from build123d import *

# Parameters (mm, degrees)
SKETCH1_R           = 2.2
SKETCH1_R_2         = 1.6
BOSS_EXTRUDE1_DEPTH = 2
SKETCH3_R           = 20.4
SKETCH3_R_2         = 20
CUT_EXTRUDE9_DEPTH  = 0.2
SKETCH6_W           = 9.4
SKETCH6_H           = 1.8
BOSS_EXTRUDE2_DEPTH = 5.2
SKETCH7_W           = 1.8
SKETCH7_H           = 9.4
BOSS_EXTRUDE3_DEPTH = 5.2
BOSS_EXTRUDE4_DEPTH = 9.4
CUT_EXTRUDE10_DEPTH = 0.6
SKETCH11_W          = 83.6
SKETCH11_H          = 59.2
CUT_EXTRUDE11_DEPTH = 0.4
BOSS_EXTRUDE5_DEPTH = 9.4
CUT_EXTRUDE12_DEPTH = 1
CUT_EXTRUDE13_DEPTH = 10
FILLET1_R           = 1
FILLET4_R           = 1
FILLET8_R           = 1
FILLET9_R           = 1
FILLET10_R          = 1


with BuildPart() as part:
    # Sketch1 → Boss-Extrude1 (new body)
    with BuildSketch(Plane(origin=(0, 0, 0), x_dir=(0, 1, 0), z_dir=(0, 0, 1))):
        with BuildLine():
            Line((65.347379442, -55.6), (-65.347379442, -55.6))
            ThreePointArc((-65.347379442, -55.6), (0, 85.8), (65.347379442, -55.6))
        make_face()
        with Locations(Location((-79.5, -5, 0), (0, 0, 270))):
            Circle(SKETCH1_R, mode=Mode.SUBTRACT)
        with Locations(Location((-79.5, 16.27256024, 0), (0, 0, 270))):
            Circle(SKETCH1_R_2, mode=Mode.SUBTRACT)
        with Locations(Location((79.5, 16.27256024, 0), (0, 0, 90))):
            Circle(SKETCH1_R_2, mode=Mode.SUBTRACT)
        with Locations(Location((79.5, -5, 0), (0, 0, 90))):
            Circle(SKETCH1_R, mode=Mode.SUBTRACT)
    extrude(amount=BOSS_EXTRUDE1_DEPTH)

    # Sketch3 → Cut-Extrude9 (cut)
    # profile 1 of 4: a face of its own
    with BuildSketch(Plane.XY.offset(2)):
        with Locations((-54.772, 35.000400226)):
            Circle(SKETCH3_R)
        with Locations((-54.772, 35.000400226)):
            Circle(SKETCH3_R_2, mode=Mode.SUBTRACT)
    # profile 2 of 4: a face of its own
    with BuildSketch(Plane.XY.offset(2)):
        with Locations(Location((-54.772, -35.000400226, 0), (0, 0, 180))):
            Circle(SKETCH3_R)
        with Locations(Location((-54.772, -35.000400226, 0), (0, 0, 180))):
            Circle(SKETCH3_R_2, mode=Mode.SUBTRACT)
    # profile 3 of 4: a face of its own
    with BuildSketch(Plane.XY.offset(2)):
        with Locations((35, -54.772255751)):
            Circle(SKETCH3_R)
        with Locations((35, -54.772255751)):
            Circle(SKETCH3_R_2, mode=Mode.SUBTRACT)
    # profile 4 of 4: a face of its own
    with BuildSketch(Plane.XY.offset(2)):
        with Locations((35, 54.772255751)):
            Circle(SKETCH3_R)
        with Locations((35, 54.772255751)):
            Circle(SKETCH3_R_2, mode=Mode.SUBTRACT)
    extrude(amount=-CUT_EXTRUDE9_DEPTH, mode=Mode.SUBTRACT)

    # Sketch6 → Boss-Extrude2 (add)
    with BuildSketch(Plane.XY.offset(2)):
        with Locations((-4.8, -69.6)):
            Rectangle(SKETCH6_W, SKETCH6_H)
        with Locations((-4.8, 69.6)):
            Rectangle(SKETCH6_W, SKETCH6_H)
    extrude(amount=BOSS_EXTRUDE2_DEPTH)

    # Sketch7 → Boss-Extrude3 (add)
    with BuildSketch(Plane.XY.offset(2)):
        with Locations((-75.6, 0)):
            Rectangle(SKETCH7_W, SKETCH7_H)
    extrude(amount=BOSS_EXTRUDE3_DEPTH)

    # Sketch8 → Boss-Extrude4 (add)
    with BuildSketch(Plane.YZ.offset(-0.1)):
        Polygon((-68.7, 7.2), (-68.7, 4.6), (-67.7, 4.6), align=None)
        Polygon((67.7, 4.6), (68.7, 7.2), (68.7, 4.6), align=None)
    extrude(amount=-BOSS_EXTRUDE4_DEPTH)

    # Sketch10 → Cut-Extrude10 (cut)
    with BuildSketch(Plane.XY.offset(2)):
        Polygon((55.6, -29.6), (-28, -29.6), (-28, 29.6), (55.6, 29.6), (55.6, 30.6), (-29, 30.6), (-29, -30.6), (55.6, -30.6), align=None)
    extrude(amount=-CUT_EXTRUDE10_DEPTH, mode=Mode.SUBTRACT)

    # Sketch11 → Cut-Extrude11 (cut)
    with BuildSketch(Plane.XY.offset(2)):
        with Locations((13.8, 0)):
            Rectangle(SKETCH11_W, SKETCH11_H)
    extrude(amount=-CUT_EXTRUDE11_DEPTH, mode=Mode.SUBTRACT)

    # Sketch13 → Boss-Extrude5 (add)
    with BuildSketch(Plane.XZ.offset(4.7)):
        Polygon((-74.7, 7.2), (-74.7, 4.6), (-73.7, 4.6), align=None)
    extrude(amount=-BOSS_EXTRUDE5_DEPTH)

    # Sketch15 → Cut-Extrude12 (cut)
    with BuildSketch(Plane(origin=(0, 0, 0), x_dir=(1, 0, 0), z_dir=(0, 0, -1))):
        with BuildLine():
            Line((-83.436442877, 20), (55.6, 20))
            Line((55.6, 20), (55.6, -20))
            Line((55.6, -20), (-83.436442877, -20))
            ThreePointArc((-83.436442877, -20), (-85.8, 0), (-83.436442877, 20))
        make_face()
    extrude(amount=-CUT_EXTRUDE12_DEPTH, mode=Mode.SUBTRACT)

    # Sketch17 → Cut-Extrude13 (cut)
    with BuildSketch(Plane.XY.offset(2)):
        Polygon((-10.9, -71.9), (-10.9, -61.9), (-11.5, -61.9), (-11.5, -72.5), (1.9, -72.5), (1.9, -61.9), (1.3, -61.9), (1.3, -71.9), align=None)
        Polygon((1.9, 72.5), (-11.5, 72.5), (-11.5, 61.9), (-10.9, 61.9), (-10.9, 71.9), (1.3, 71.9), (1.3, 61.9), (1.9, 61.9), align=None)
        Polygon((-78.5, 6.7), (-78.5, -6.7), (-67.9, -6.7), (-67.9, -6.1), (-77.9, -6.1), (-77.9, 6.1), (-67.9, 6.1), (-67.9, 6.7), align=None)
    extrude(amount=-CUT_EXTRUDE13_DEPTH, mode=Mode.SUBTRACT)

    # Fillet1
    fillet1_edges = [part.edges().sort_by_distance(p)[0] for p in [
        (-10.9, -71.9, 1),
    ]]
    fillet(fillet1_edges, radius=FILLET1_R)

    # Fillet4
    # the kernel refuses this fillet: 1 mm, written as the material it adds along each edge
    with BuildSketch(Plane(origin=(1.3, -61.9, 2), x_dir=(0, -1, 0), z_dir=(0, 0, -1))) as fillet4_piece_1:
        with BuildLine():
            CenterArc((0.916515139, -1), FILLET4_R, 90, 66.421821522)
            Line((0, -0.6), (0, 0))
            Line((0, 0), (0.916515139, 0))
        make_face()
    extrude(amount=2)
    # the kernel refuses this fillet: 1 mm, written as the material it takes off along each edge
    with BuildSketch(Plane(origin=(1.3, -71.9, 4.5), x_dir=(-1, 0, 0), z_dir=(0, 0, -1))) as fillet4_2_piece_1:
        with BuildLine():
            CenterArc((FILLET4_R, FILLET4_R), FILLET4_R, 180, 90)
            Line((0, FILLET4_R), (0, 0))
            Line((0, 0), (FILLET4_R, 0))
        make_face()
    extrude(amount=7, mode=Mode.SUBTRACT)

    # Fillet8
    # the kernel refuses this fillet: 1 mm, written as the material it adds along each edge
    with BuildSketch(Plane(origin=(-10.9, -61.9, 2), x_dir=(0, -1, 0), z_dir=(0, 0, -1))) as fillet8_piece_1:
        with BuildLine():
            CenterArc((0.916515139, 1), FILLET8_R, 203.578178478, 66.421821522)
            Line((0, 0.6), (-0.018330303, 0.592))
            ThreePointArc((-0.018330303, 0.592), (-0.02, 0.3), (-0.02, 0))
            Line((-0.02, 0), (0, -0.02))
            Line((0, -0.02), (0.916515139, -0.02))
            Line((0.916515139, -0.02), (0.916515139, 0))
        make_face()
    extrude(amount=2)

    # Fillet9
    # the kernel refuses this fillet: 1 mm, written as the material it adds along each edge
    with BuildSketch(Plane(origin=(-10.9, 61.9, 2), x_dir=(-1, 0, 0), z_dir=(0, 0, -1))) as fillet9_piece_1:
        with BuildLine():
            CenterArc((1, 0.916515139), FILLET9_R, 180, 66.421821522)
            Line((0, 0.916515139), (0, 0))
            Line((0, 0), (0.6, 0))
        make_face()
    extrude(amount=2)
    with BuildSketch(Plane(origin=(1.3, 61.9, 2), x_dir=(1, 0, 0), z_dir=(0, 0, -1))) as fillet9_piece_2:
        with BuildLine():
            CenterArc((1, -0.916515139), FILLET9_R, 113.578178478, 66.421821522)
            Line((0, -0.916515139), (0, 0))
            Line((0, 0), (0.6, 0))
        make_face()
    extrude(amount=2)
    # the kernel refuses this fillet: 1 mm, written as the material it takes off along each edge
    with BuildSketch(Plane(origin=(1.3, 71.9, 4.5), x_dir=(0, -1, 0), z_dir=(0, 0, -1)), Plane(origin=(-10.9, 71.9, 4.5), x_dir=(1, 0, 0), z_dir=(0, 0, -1))) as fillet9_2_piece_1:
        with BuildLine():
            CenterArc((FILLET9_R, FILLET9_R), FILLET9_R, 180, 90)
            Line((0, FILLET9_R), (0, 0))
            Line((0, 0), (FILLET9_R, 0))
        make_face()
    extrude(amount=7, mode=Mode.SUBTRACT)

    # Fillet10
    # the kernel refuses this fillet: 1 mm, written as the material it adds along each edge
    with BuildSketch(Plane(origin=(-67.9, -6.1, 2), x_dir=(0, -1, 0), z_dir=(0, 0, -1))) as fillet10_piece_1:
        with BuildLine():
            CenterArc((1, 0.916515139), FILLET10_R, 180, 66.421821522)
            Line((0, 0.916515139), (0, 0))
            Line((0, 0), (0.6, 0))
        make_face()
    extrude(amount=1)
    with BuildSketch(Plane(origin=(-67.9, 6.1, 2), x_dir=(0, 1, 0), z_dir=(0, 0, -1))) as fillet10_piece_2:
        with BuildLine():
            CenterArc((1, -0.916515139), FILLET10_R, 113.578178478, 66.421821522)
            Line((0, -0.916515139), (0, 0))
            Line((0, 0), (0.6, 0))
        make_face()
    extrude(amount=1)
    # the kernel refuses this fillet: 1 mm, written as the material it takes off along each edge
    with BuildSketch(Plane(origin=(-77.9, -6.1, 4.5), x_dir=(1, 0, 0), z_dir=(0, 0, -1))) as fillet10_2_piece_1:
        with BuildLine():
            CenterArc((FILLET10_R, -FILLET10_R), FILLET10_R, 90, 90)
            Line((0, -FILLET10_R), (0, 0))
            Line((0, 0), (FILLET10_R, 0))
        make_face()
    extrude(amount=6, mode=Mode.SUBTRACT)
    with BuildSketch(Plane(origin=(-77.9, 6.1, 4.5), x_dir=(1, 0, 0), z_dir=(0, 0, -1))) as fillet10_2_piece_2:
        with BuildLine():
            CenterArc((FILLET10_R, FILLET10_R), FILLET10_R, 180, 90)
            Line((0, FILLET10_R), (0, 0))
            Line((0, 0), (FILLET10_R, 0))
        make_face()
    extrude(amount=6, mode=Mode.SUBTRACT)


solid = part.part
Build history of the part. All positions in model axes, mm. A direction names the side the tool comes from. Round coordinates to 2 decimals unless told otherwise and drop trailing zeros. Loops run counter-clockwise (first coordinate to the right, second up) from the corner with the lowest first, then second, coordinate; pieces in that order, holes last. Notation, with made-up numbers: (-3.75, 43.5) -> (12.25, 43.5) arc R7 cw to (12.25, 48.5) -> close; hole circle Ø1 at (45.5, 54.5). An arc over 180 degrees is marked (long way). Answer in a Markdown table with one row per item.
Item 1: Saw through at A-A (y = 0). Write the cut outline in (x, z), and give its area (3 significant figures).
Answers below:
| item | result |
|---|---|
| outline | (-85.8, 1) -> (-78.5, 1) -> (-78.5, 2) -> (-85.8, 2) -> close; (-77.9, 1) -> (55.6, 1) -> (55.6, 1.6) -> (-28, 1.6) -> (-28, 1.4) -> (-29, 1.4) -> (-29, 2) -> (-74.7, 2) -> (-74.7, 4.6) -> (-73.7, 4.6) -> (-74.7, 7.2) -> (-76.5, 7.2) -> (-76.5, 2) -> (-77.9, 2) -> close |
| area | 117 mm² |
Item 2: Pin check, flat tips, straight feed: pin 1 (5 mm diameter, centred on x = 19, y = -6, fed in from +Z); pin 2 (2 mm diameter, centred on y = -69.5, z = 6, fed in from -X); pin 3 (2 mm diameter, centred on y = -69, z = 1, fed in from +X); pin 4 (1.9 mm diameter, centred on x = -16.27, y = -79.5, fed in from +Z). Stop position of each tip, or through.
Answers below:
| item | result |
|---|---|
| pin 1 | stops at z = 1.6 |
| pin 2 | stops at x = -9.5 |
| pin 3 | stops at x = 52.32 |
| pin 4 | passes through |
Item 3: Saw through at D-D (x = -23). Write the cut outline in (y, z), and give its area (3 significant figures).
Answers below:
| item | result |
|---|---|
| outline | (-82.66, 0) -> (-20, 0) -> (-20, 1) -> (20, 1) -> (20, 0) -> (82.66, 0) -> (82.66, 2) -> (30.6, 2) -> (30.6, 1.4) -> (29.6, 1.4) -> (29.6, 1.6) -> (-29.6, 1.6) -> (-29.6, 1.4) -> (-30.6, 1.4) -> (-30.6, 2) -> (-82.66, 2) -> close |
| area | 266 mm² |
Item 4: Saw through at C-C (x = 5). Write the cut outline in (y, z).
Answers below:
| item | result |
|---|---|
| outline | (-85.65, 0) -> (-81.7, 0) -> (-81.7, 2) -> (-85.65, 2) -> close; (-77.3, 0) -> (-20, 0) -> (-20, 1) -> (20, 1) -> (20, 0) -> (77.3, 0) -> (77.3, 2) -> (30.6, 2) -> (30.6, 1.4) -> (29.6, 1.4) -> (29.6, 1.6) -> (-29.6, 1.6) -> (-29.6, 1.4) -> (-30.6, 1.4) -> (-30.6, 2) -> (-77.3, 2) -> close; (81.7, 0) -> (85.65, 0) -> (85.65, 2) -> (81.7, 2) -> close |
Item 5: Which spindle directions (+Z, -Z, +X, -X, +Y, -Y) get a long thin tool onto all of the face, cutting with end or side? Do faces 4 (the cylindrical face through (6.183, -77.645, 0.986)), 5 (the flat face through (-39.8, 21.5, 1.8)), 6 (the flat face through (13, 0, 1.6)), 7 (the flat face through (-76.5, 0, 5)), 8 (the flat face through (-55, 35, 2)). Say none if no direction does.
Answers below:
| item | result |
|---|---|
| face 4 | +Z, -Z |
| face 5 | +Z |
| face 6 | +Z, +X |
| face 7 | +Z, -X, +Y, -Y |
| face 8 | +Z, +X, -X, +Y, -Y |
Item 6: Drill centre lines: L1, parallel to Y at x = -3, z = 1.25; L2, parallel to Y at x = 35, z = 1.95; L3, parallel to X at y = 69.5, z = 1. Where is each one in solid material? Low to high. Write a range as [from, to].
Answers below:
| item | result |
|---|---|
| L1 | y = [-85.75, -72.5], [-71.9, 71.9], [72.5, 85.75] |
| L2 | y = [-78.34, -75.17], [-74.77, -34.77], [-34.37, -30.6], [30.6, 34.37], [34.77, 74.77], [75.17, 78.34] |
| L3 | x = [-50.31, -11.5], [-10.9, 1.3], [1.9, 50.31] |
Item 7: Mould opens along Y. For faces 1 (the flat face through (35, -54, 2)), 2 (the flat face through (-69.8, -21.5, 1.8)), 3 (the flat face through (-5, -70.5, 5)) say: +Y half, -Y half, draft (parallel to the pull), parting line (faces both ways), or undercut.
Answers below:
| item | result |
|---|---|
| face 1 | draft |
| face 2 | undercut |
| face 3 | -Y half |
Item 8: Saw through at B-B (z = 3.25). Write the cut outline in (x, y), and give its area (3 significant figures).
Answers below:
| item | result |
|---|---|
| outline | (-76.5, -4.7) -> (-74.7, -4.7) -> (-74.7, 4.7) -> (-76.5, 4.7) -> close; (-9.5, -70.5) -> (-0.1, -70.5) -> (-0.1, -68.7) -> (-9.5, -68.7) -> close; (-9.5, 68.7) -> (-0.1, 68.7) -> (-0.1, 70.5) -> (-9.5, 70.5) -> close |
| area | 50.8 mm² |
